from build123d import *

# Parameters (mm, degrees)
F0_R     = 3.625
F1_DEPTH = 2.75
F2_R     = 0.5
F3_T     = -1.25
F5_DEPTH = 1.5


with BuildPart() as f1:
    # F0 (on Right) → F1 (new body, symmetric)
    with BuildSketch(Plane.YZ):
        Circle(F0_R)
    extrude(amount=F1_DEPTH, both=True)

    # F2
    f2_edges = [f1.edges().sort_by_distance(p)[0] for p in [
        (2.75, -3.625, 0),
    ]]
    fillet(f2_edges, radius=F2_R)

    # F3
    f3_openings = [f1.faces().sort_by_distance(p)[0] for p in [
        (-2.75, 0, 0),
    ]]
    offset(amount=F3_T, openings=f3_openings)

    # F4 (on face) → F5 (join)
    with BuildSketch(Plane(origin=(-2.75, 0, 0), x_dir=(0, -1, 0), z_dir=(-1, 0, 0))):
        with BuildLine():
            Line((3.546565, -0.75), (5.046565, -0.75))
            Line((5.046565, -0.75), (5.046565, 0.75))
            Line((5.046565, 0.75), (3.546565, 0.75))
            ThreePointArc((3.546565, 0.75), (3.625, 0), (3.546565, -0.75))
        make_face()
        with BuildLine():
            Line((-3.546565, 0.75), (-5.046565, 0.75))
            Line((-5.046565, 0.75), (-5.046565, -0.75))
            Line((-5.046565, -0.75), (-3.546565, -0.75))
            ThreePointArc((-3.546565, -0.75), (-3.625, 0), (-3.546565, 0.75))
        make_face()
    extrude(amount=-F5_DEPTH)


solid = f1.part
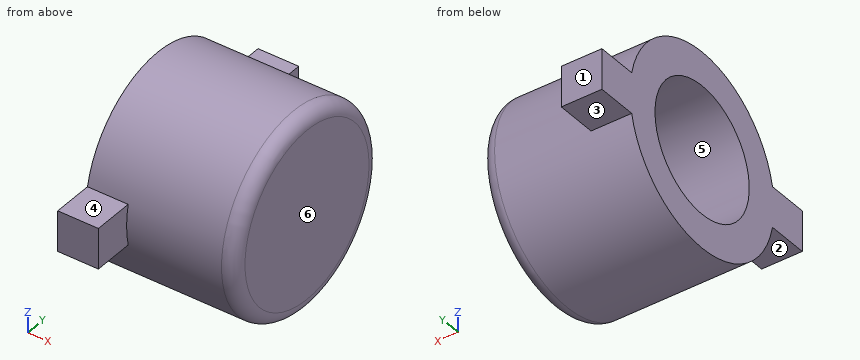
Design review of the part built by this model. Coordinates are the model's own, in mm. Face numbers are marked on the shaded views. A direction names the side the tool comes from. Give positions to 0.01 mm unless a question says otherwise; leave off trailing zeros. Loops run counter-clockwise (first coordinate to the right, second up) from the corner with the lowest first, then second, coordinate; pieces in that order, holes last. Notation, with made-up numbers: (35.5, -22.5) - (48.5, -22.5) arc R24 ccw to (48.5, 14.5) - close; hole circle Ø11 at (-20.75, 33). An arc over 180 degrees is marked (long way). Write item = value, one per line.
1) Tool access review of the marked faces 1 and 2: name each direction out of +Z, -Z, +X, -X, +Y, -Y from which nothing blocks a thin tool from reaching the whole face with its end or side.
Result sheet:
face_1 = +Z, -Z, +X, -X, +Y
face_2 = -Z, +X, -X, -Y
2) Take a section at A-A on y = 0. State the section outline as (x, z) points (3 decimals), and give its area (3 significant figures).
Result sheet:
outline = (-2.75, -3.625) - (2.25, -3.625) arc R0.5 ccw to (2.75, -3.125) - (2.75, 3.125) arc R0.5 ccw to (2.25, 3.625) - (-2.75, 3.625) - (-2.75, 2.375) - (1.5, 2.375) - (1.5, -2.375) - (-2.75, -2.375) - close
area = 19.6 mm2
3) Take a section at B-B on z = 0. State the section outline as (x, y) points (3 decimals), and give its area (3 significant figures).
Result sheet:
outline = (-2.75, -5.047) - (-1.25, -5.047) - (-1.25, -3.625) - (2.25, -3.625) arc R0.5 ccw to (2.75, -3.125) - (2.75, 3.125) arc R0.5 ccw to (2.25, 3.625) - (-1.25, 3.625) - (-1.25, 5.047) - (-2.75, 5.047) - (-2.75, 2.375) - (1.5, 2.375) - (1.5, -2.375) - (-2.75, -2.375) - close
area = 23.8 mm2
4) Clearance check with flat-ended pins moving along their axes: pin 1 Ø1.6 at (y, z) = (-4.5, 0) entering from +X; pin 2 Ø1.6 at (x, y) = (-2, -4.5) entering from +Z; pin 3 Ø1.6 at (x, y) = (-2, 4) entering from -Z. State where each tip first meets the part, or that it passes through.
Result sheet:
pin_1 = -1.25
pin_2 = 0.75
pin_3 = -1.7
5) To check wall thickness, follow line 1 (Z direction, x = -1.75, y = 0) (3 decimals); line 2 (X direction, y = 0.25, z = 0.5); line 3 (Y direction, x = -2.35, z = 1.5). State the ranges of each line that lie inside material, in increasing order.
Result sheet:
line_1 = -3.625 to -2.375, 2.375 to 3.625
line_2 = 1.5 to 2.75
line_3 = -3.3 to -1.84, 1.84 to 3.3
6) Take a section at C-C on x = -0.3. State the section outline as (y, z) points (3 decimals), and give its area (3 significant figures).
Result sheet:
outline = circle Ø7.25 at (0, 0); hole circle Ø4.75 at (0, 0)
area = 23.6 mm2
7) Draft analysis for pull direction Z (two halves, no side actions). For the marked faces 3, 4, 5 and 6, state which applies: +Z half, -Z half, draft (parallel to the pull), parting line (faces both ways), or undercut.
Result sheet:
face_3 = -Z half
face_4 = +Z half
face_5 = undercut
face_6 = draft
